Check sheet for the drawn part. Datum: minimum x, y, z corner. Units: mm. A direction names the side the tool comes from. Coordinates: 2 decimals unless noted, no trailing zeros. Write each loop counter-clockwise with the first axis right and the second up, starting at its lowest first coordinate (ties: lowest second). Pieces come first, ordered by that corner, then holes. Notation, with made-up numbers: (-3.75, -37) - (14.25, -37) arc R23 cw to (14.25, 1) - close; hole circle Ø6 at (74, 37.5). An arc over 180 degrees is marked (long way). Answer as CSV lines item,"result". Start each with the question number.
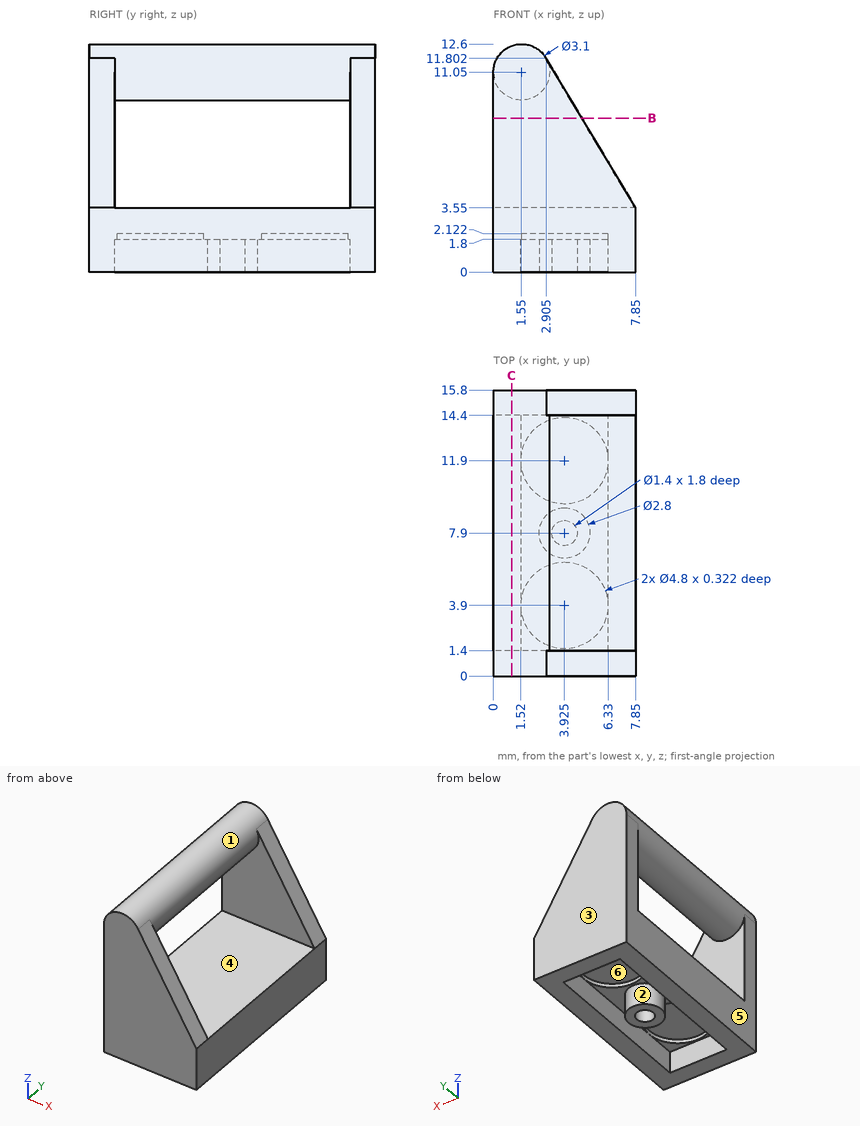
(1) Release check for a two-part mould opening along X. For the marked faces 4, 5 and 6 record: pulls with the +X half, pulls with the -X half, needs draft (parallel to the pull), parting line crosses it, or undercut.
(2) Cross-section at C-C on x = 1. Record the boundary of the cut face in (y, z).
(3) Go/stop test with a flat-tipped pin: P1, Ø4, axis at x = 3.925, y = 11.9, coming from the +Z side. Record where the tip stops, or that it passes through.
(4) Cross-section at B-B on z = 8.5. Record the boundary of the cut face in (x, y).
(5) Tool access check on the marked faces 1, 2 and 3. Record the directions out of +Z, -Z, +X, -X, +Y, -Y that give a thin tool (end or side, any length) a straight path to the whole face; none if there is none.
(6) Material ranges on probe 1 along Y at (x, z) = (4, 1.25) (1 decimal); probe 2 along Y at (x, z) = (6, 5.25); probe 3 along Y at (x, z) = (4.25, 1.5), recorded low to high. Write a range as from..to.
Checked values:
1,face 4,"needs draft"
1,face 5,"pulls with the -X half"
1,face 6,"undercut"
2,outline,"(0, 0) - (15.8, 0) - (15.8, 12.5) - (0, 12.5) - close; hole (1.4, 3.55) - (14.4, 3.55) - (14.4, 9.6) - (1.4, 9.6) - close"
3,P1,"z = 12.55"
4,outline,"(0, 0) - (4.88, 0) - (4.88, 1.4) - (0, 1.4) - close; (0, 14.4) - (4.88, 14.4) - (4.88, 15.8) - (0, 15.8) - close"
5,face 1,"none"
5,face 2,"-Z"
5,face 3,"+Z, -Z, +X, -X, +Y"
6,probe 1,"0..1.4, 6.5..7.2, 8.6..9.3, 14.4..15.8"
6,probe 2,"0..1.4, 14.4..15.8"
6,probe 3,"0..1.4, 6.54..7.28, 8.52..9.26, 14.4..15.8"
